from build123d import *

# Parameters (mm, degrees)
F0_W     = 94.4796726108
F0_H     = 86.6620987654
F1_DEPTH = 54.864
F3_DEPTH = 94.4806726108
F4_R     = 14.2396166793
F5_DEPTH = 25.4


with BuildPart() as f1:
    # F0 (on Top) → F1 (new body)
    with BuildSketch(Plane.XY):
        with Locations((-1.709651202, -1.7030909657)):
            Rectangle(F0_W, F0_H)
    extrude(amount=F1_DEPTH)

    # F2 (on face) → F3 (cut, through all)
    with BuildSketch(Plane.YZ.offset(45.5301851034)):
        Polygon((-36.2590327859, 15.8963445574), (-15.7042443752, 0), (25.5974382162, 0), (25.5974382162, 15.8963445574), align=None)
    extrude(amount=-F3_DEPTH, mode=Mode.SUBTRACT)

    # F4 (on face) → F5 (join)
    with BuildSketch(Plane.XY.offset(54.864)):
        Circle(F4_R)
    extrude(amount=F5_DEPTH)


solid = f1.part
Work out the finished part from the listing and answer in its coordinate system (mm). A direction names the side the tool comes from. Round coordinates to 2 decimals unless told otherwise and drop trailing zeros. Write each loop counter-clockwise with the first axis right and the second up, starting at its lowest first coordinate (ties: lowest second). Pieces come first, ordered by that corner, then holes.
1) Straight lines are drawn through the part: line 1 (Z direction, x = -26, y = -41); line 2 (Z direction, x = -11, y = -10.5); line 3 (Y direction, x = 28.5, z = 11.5). For each, find the intervals that lie inside material, in ascending order.
2) A tool of negligible diameter and unlimited length cuts with its end or side. For faces 4 (the flat face through (-13, -11, 54.864)), 5 (the flat face through (-1.048, -26.126, 8.059)), 6 (the flat face through (-48.949, -2, 33)), 7 (the flat face through (-2, 34, 0)), 8 (the flat face through (-1, 25.597, 8)), from which of +Z, -Z, +X, -X, +Y, -Y can it reach the whole face along a straight path? Write none if from no direction.
3) A cutting plane is placed at D-D (x = 0). Give the vertices of the cut face in (y, z).
4) A cutting plane is placed at A-A (x = 19.5). Give the vertices of the cut face in (y, z).
5) A cutting plane is placed at C-C (y = -18). Give the vertices of the cut face in (x, z), plus the area to 3 significant figures.
6) A cutting plane is placed at B-B (y = 0). Give the vertices of the cut face in (x, z).
7) The mould has two halves that part along Y. Classify faces 1 (the flat face through (-1, -5, 15.896)), 2 (the flat face through (45.53, -2, 33)), 3 (the cylindrical face through (-11.3, -8.665, 67.386)): pulls with the +Y half, pulls with the -Y half, needs draft (parallel to the pull), parting line crosses it, or undercut.
8) Given pin 1 Ø5 at (x, y) = (32, 0) entering from -Z; pin 2 Ø10 at (y, z) = (-6, 71.5) entering from -X, each flat-ended and moving along its own axis, determine where each tip first touches the part or whether it passes through.
Completed:
1. line 1: z = 0 to 54.86
1. line 2: z = 15.9 to 54.86
1. line 3: y = -45.03 to -30.57, 25.6 to 41.63
2. face 4: +Z
2. face 5: +X, -X
2. face 6: +Z, -Z, -X, +Y, -Y
2. face 7: -Z, +X, -X, +Y, -Y
2. face 8: -Z, +X, -X
3. outline: (-45.03, 0) - (-15.7, 0) - (-36.26, 15.9) - (25.6, 15.9) - (25.6, 0) - (41.63, 0) - (41.63, 54.86) - (14.24, 54.86) - (14.24, 80.26) - (-14.24, 80.26) - (-14.24, 54.86) - (-45.03, 54.86) - close
4. outline: (-45.03, 0) - (-15.7, 0) - (-36.26, 15.9) - (25.6, 15.9) - (25.6, 0) - (41.63, 0) - (41.63, 54.86) - (-45.03, 54.86) - close
5. outline: (-48.95, 0) - (45.53, 0) - (45.53, 1.78) - (-48.95, 1.78) - close; (-48.95, 15.9) - (45.53, 15.9) - (45.53, 54.86) - (-48.95, 54.86) - close
5. area: 3,850 mm2
6. outline: (-48.95, 15.9) - (45.53, 15.9) - (45.53, 54.86) - (14.24, 54.86) - (14.24, 80.26) - (-14.24, 80.26) - (-14.24, 54.86) - (-48.95, 54.86) - close
7. face 1: undercut
7. face 2: needs draft
7. face 3: parting line crosses it
8. pin 1: stops at z = 15.9
8. pin 2: stops at x = -14.2
